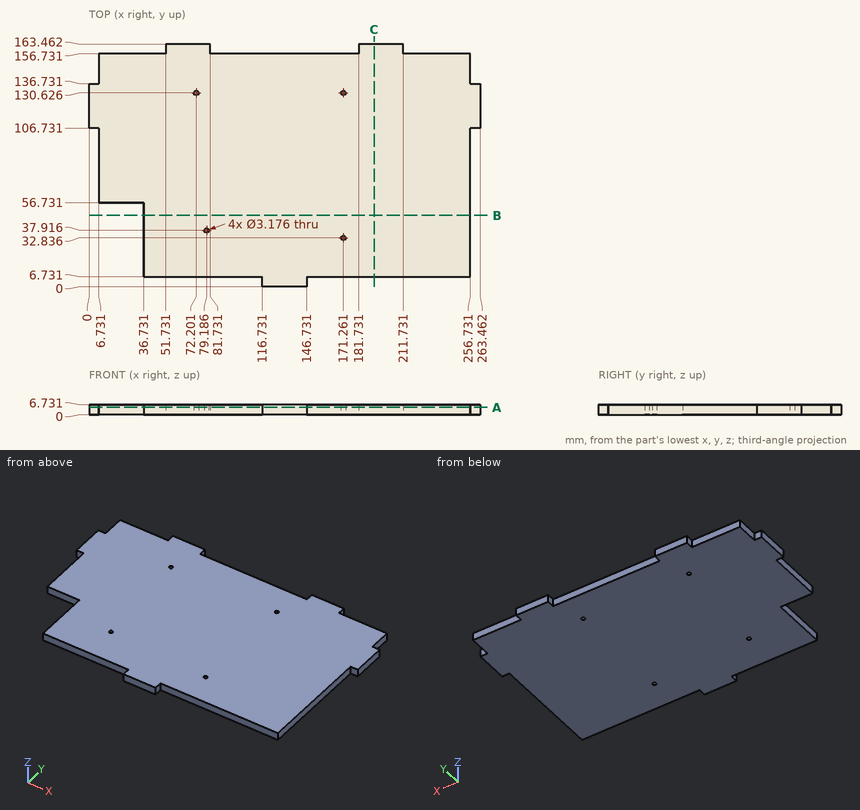
Here's the drawing with two shaded views (mm, measured from the low corner). I have some questions. Give positions to 0.01 mm unless a question says otherwise; leave off trailing zeros. Order: outer loops, then holes, each group sorted by start corner. A loop starts at its lowest first (then second) coordinate and runs counter-clockwise, first axis right, second up.
Q1. Suppose I cut it at C-C, the plane x = 192. Write out the boundary of the cut face in (y, z).
Q2. I'm going to push flat-ended pins straight in: P1, Ø3.5, axis at x = 241, z = 2, coming from the +Y side; P2, Ø2, axis at y = 160.5, z = 4, coming from the -X side; P3, Ø1.5, axis at y = 70, z = 1, coming from the +X side. Where does each tip first touch, or does it pass through?
Q3. If I drill on line 1 along X through (y, z) = (131, 1); line 2 along X through (y, z) = (129.5, 2); line 3 along Y through (x, z) = (31.5, 0.5), over which ranges is the centre line in solid material (lowest first)?
Q4. Suppose I cut it at A-A, the plane z = 5. Count the separate pieces of the cut face and the enclosed holes in it, and give its area (3 significant figures).
Q5. Suppose I cut it at B-B, the plane y = 48. Write out the boundary of the cut face in (x, z).
Solution:
1. outline: (6.73, 0) - (163.46, 0) - (163.46, 6.73) - (6.73, 6.73) - close
2. P1: stops at y = 156.73
2. P2: stops at x = 51.73
2. P3: stops at x = 256.73
3. line 1: x = 0 to 70.66, 73.74 to 169.72, 172.8 to 263.46
3. line 2: x = 0 to 71.08, 73.32 to 170.14, 172.38 to 263.46
3. line 3: y = 56.73 to 156.73
4. separate pieces: 1
4. enclosed holes: 4
4. area: 37,000 mm2
5. outline: (36.73, 0) - (256.73, 0) - (256.73, 6.73) - (36.73, 6.73) - close
